The model under review builds one solid part; all positions refer to its coordinate system, in mm. A direction names the side the tool comes from. Give positions to 0.01 mm unless a question says otherwise; leave off trailing zeros. Loops run counter-clockwise (first coordinate to the right, second up) from the corner with the lowest first, then second, coordinate; pieces in that order, holes last. Notation, with made-up numbers: M 49.5,70.5 L 107.5,70.5 A22 ccw 107.5,79.5 Z; hole C 81,88.5 d7. An arc over 180 degrees is marked long. Put each result on its own line as item: value. Start each with the question number.
from build123d import *

# Parameters (mm, degrees)
SKETCH1_W                               = 26
SKETCH1_H                               = 10
SKETCH1_R                               = 1.5
BOSS_EXTRUDE5_DEPTH                     = 3.302
CROQUIS7_W                              = 12
CROQUIS7_H                              = 8
SALIENTE_EXTRUIR2_DEPTH                 = 10
TALADRO_DE_MARGEN_PARA_1_43_D           = 6.7564
TALADRO_DE_MARGEN_PARA_1_43_CSINK_D     = 8.0264
TALADRO_DE_MARGEN_PARA_1_43_CSINK_ANGLE = 82
CROQUIS13_R                             = 1.5
CORTAR_EXTRUIR3_DEPTH                   = 3


with BuildPart() as part:
    # Sketch1 → Boss-Extrude5 (new body)
    with BuildSketch(Plane(origin=(0, 0, 0), x_dir=(1, 0, 0), z_dir=(0, 1, 0))):
        Rectangle(SKETCH1_W, SKETCH1_H)
        with Locations(Location((-9.9, 0, 0), (0, 0, 90))):
            Circle(SKETCH1_R, mode=Mode.SUBTRACT)
        with Locations(Location((9.9, 0, 0), (0, 0, 90))):
            Circle(SKETCH1_R, mode=Mode.SUBTRACT)
    extrude(amount=BOSS_EXTRUDE5_DEPTH)

    # Croquis7 → Saliente-Extruir2 (add)
    with BuildSketch(Plane(origin=(0, 3.302, 0), x_dir=(1, 0, 0), z_dir=(0, 1, 0))):
        Rectangle(CROQUIS7_W, CROQUIS7_H)
    extrude(amount=SALIENTE_EXTRUIR2_DEPTH)

    # Taladro de margen para 1/43 (through all)
    with Locations(Plane.XY.offset(4)):
        with Locations((0, 8.302)):
            CounterSinkHole(TALADRO_DE_MARGEN_PARA_1_43_D / 2, TALADRO_DE_MARGEN_PARA_1_43_CSINK_D / 2, counter_sink_angle=TALADRO_DE_MARGEN_PARA_1_43_CSINK_ANGLE)

    # Croquis13 → Cortar-Extruir3 (cut)
    with BuildSketch(Plane(origin=(0, 13.302, 0), x_dir=(1, 0, 0), z_dir=(0, 1, 0))):
        with Locations(Location((0, 0, 0), (0, 0, 270))):
            Circle(CROQUIS13_R)
    extrude(amount=-CORTAR_EXTRUIR3_DEPTH, mode=Mode.SUBTRACT)


solid = part.part
(1) We need section D-D, the plane x = 0. Write out the cut boundary in (y, z), plus the area to 3 significant figures.
(2) We need section A-A, the plane z = 0. Write out the cut boundary in (x, y).
(3) Draft analysis for pull direction Z (two halves, no side actions). For faces 4 (the flat face through (13, 2, 0)), 5 (the cylindrical face through (-11.387, 1.628, 0.195)), 6 (the flat face through (0, 2, -5)), state which applies: +Z half, -Z half, draft (parallel to the pull), parting line (faces both ways), or undercut.
(4) Insertion check: pin 1 (3 mm diameter, centred on x = 10.5, y = 4, fed in from -Z); pin 2 (2.5 mm diameter, centred on y = 7.5, z = -2, fed in from +X); pin 3 (4 mm diameter, centred on y = 10, z = -1.5, fed in from -X); pin 4 (5 mm diameter, centred on x = 2.5, y = 7, fed in from +Z). Each pin has a flat end and moves straight along its axis. Give the tip position at first contact, or say it passes through.
(5) We need section B-B, the plane x = -9.9. Write out the cut boundary in (y, z), plus the area to 3 significant figures.
(6) To check wall thickness, follow L1, parallel to X at y = 1.9, z = 0; L2, parallel to X at y = 12.5, z = 0; L3, parallel to Z at x = 9.9, y = 2.55. State the ranges of each line that lie inside material, in increasing order. Write a range as [from, to].
(7) For faces 1 (the flat face through (6, 8, 0)), 2 (the cylindrical face through (-0.575, 12.329, 1.386)), 3 (the flat face through (-6, 8, 0)), list the 3-axis set-ups (+Z, -Z, +X, -X, +Y, -Y) from which the entire face can be reached by the end or side of a thin tool; tool diameter is ignored.
(8) We need section C-C, the plane y = 2.75. Write out the cut boundary in (x, z), plus the area to 3 significant figures.
Check sheet entries:
1. outline: M 0,-5 L 3.3,-5 L 3.3,-4 L 4.92,-4 L 4.92,3.27 L 4.29,4 L 3.3,4 L 3.3,5 L 0,5 Z; M 11.68,-4 L 13.3,-4 L 13.3,-1.5 L 11.68,-1.5 Z; M 11.68,1.5 L 13.3,1.5 L 13.3,4 L 12.32,4 L 11.68,3.27 Z
1. area: 53.6 mm²
2. outline: M -13,0 L -11.4,0 L -11.4,3.3 L -13,3.3 Z; M -8.4,0 L 8.4,0 L 8.4,3.3 L 6,3.3 L 6,13.3 L 1.5,13.3 L 1.5,11.33 A3.38 cw long -1.5,11.33 L -1.5,13.3 L -6,13.3 L -6,3.3 L -8.4,3.3 Z; M 11.4,0 L 13,0 L 13,3.3 L 11.4,3.3 Z
3. face 4: draft
3. face 5: undercut
3. face 6: -Z half
4. pin 1: stops at z = -5
4. pin 2: stops at x = 6
4. pin 3: stops at x = -6
4. pin 4: stops at z = 4
5. outline: M 0,-5 L 3.3,-5 L 3.3,-1.5 L 0,-1.5 Z; M 0,1.5 L 3.3,1.5 L 3.3,5 L 0,5 Z
5. area: 23.1 mm²
6. L1: x = [-13, -11.4], [-8.4, 8.4], [11.4, 13]
6. L2: x = [-6, -1.5], [1.5, 6]
6. L3: z = [-5, -1.5], [1.5, 5]
7. face 1: +Z, -Z, +X, +Y
7. face 2: +Y
7. face 3: +Z, -Z, -X, +Y
8. outline: M -13,-5 L 13,-5 L 13,5 L -13,5 Z; hole C -9.9,0 d3; hole C 9.9,0 d3
8. area: 246 mm²
